from build123d import *

# Parameters (mm, degrees)
F0_W     = 10
F0_H     = 10
F3_DEPTH = 5
F1_W     = 10
F1_H     = 10
F4_DEPTH = 5
F2_W     = 10
F2_H     = 10
F5_DEPTH = 5


with BuildPart() as f3:
    # F0 (on Front) → F3 (new body, symmetric)
    with BuildSketch(Plane.XZ):
        Rectangle(F0_W, F0_H)
        Polygon((-4, 0), (0, 4), (4, 0), (0, -4), align=None, mode=Mode.SUBTRACT)
    extrude(amount=F3_DEPTH, both=True)

    # F1 (on Right) → F4 (intersect, symmetric)
    with BuildSketch(Plane.YZ):
        Rectangle(F1_W, F1_H)
        Polygon((-4, 0), (0, 4), (4, 0), (0, -4), align=None, mode=Mode.SUBTRACT)
    extrude(amount=F4_DEPTH, both=True, mode=Mode.INTERSECT)

    # F2 (on Top) → F5 (intersect, symmetric)
    with BuildSketch(Plane.XY):
        Rectangle(F2_W, F2_H)
        Polygon((-4, 0), (0, 4), (4, 0), (0, -4), align=None, mode=Mode.SUBTRACT)
    extrude(amount=F5_DEPTH, both=True, mode=Mode.INTERSECT)


solid = f3.part
Geometry check sheet. Reference: the model listing, model coordinates, mm. A direction names the side the tool comes from. Give positions to 0.01 mm unless a question says otherwise; leave off trailing zeros. Loops run counter-clockwise (first coordinate to the right, second up) from the corner with the lowest first, then second, coordinate; pieces in that order, holes last. Notation, with made-up numbers: M 73,41 L 131,41 A21 ccw 131,76 Z; hole C 34,-17 d5. An arc over 180 degrees is marked long. Answer as a JSON object with one key per item and string values. Group by question number.
Item 1: Sectioned sample at B-B on x = 0.25. Record the boundary of the cut face in (y, z).
Item 2: Sectioned sample at A-A on z = -2.5. Record the boundary of the cut face in (x, y), plus the area to 3 significant figures.
Item 3: Sectioned sample at D-D on y = 4.25. Record the boundary of the cut face in (x, z), plus the area to 3 significant figures.
Item 4: Sectioned sample at C-C on y = -1.5. Record the boundary of the cut face in (x, z).
Item 5: Material ranges on L1, parallel to Z at x = -4, y = 2; L2, parallel to Z at x = -3, y = -4.5, recorded low to high.
Item 6: Mould release check, pull along Z, two halves, no side actions. Record for faces 1 (the flat face through (-2, 4, -2)), 2 (the flat face through (-2.3, -2.3, -5)), 3 (the flat face through (-5, -2.3, -2.3)), 4 (the flat face through (4, 2, 2)): pulls with the +Z half, pulls with the -Z half, needs draft (parallel to the pull), parting line crosses it, or undercut.
Item 7: Gauge pin test, flat ends, axial feed: pin 1 (1.5 mm diameter, centred on x = 1, z = 2, fed in from -Y); pin 2 (1 mm diameter, centred on x = -1, z = 2, fed in from -Y). Record the tip position at first contact, or that the pin passes through.
Item 8: Access from +Z, -Z, +X, -X, +Y, -Y to the whole of each face (thin tool, end or side, straight path). Record for faces 5 (the flat face through (-2.3, -5, 2.3)), 6 (the flat face through (2, -4, 2)), 7 (the flat face through (2, 2, -4)), 8 (the flat face through (4, 2, -2)).
Findings below:
{
 "1": {"outline": "M -5,-5 L -3.75,-5 L -3.75,-3.75 L -5,-3.75 Z; M -5,3.75 L -3.75,3.75 L -3.75,5 L -5,5 Z; M 3.75,-5 L 5,-5 L 5,-3.75 L 3.75,-3.75 Z; M 3.75,3.75 L 5,3.75 L 5,5 L 3.75,5 Z"},
 "2": {"outline": "M -5,-5 L -1.5,-5 L -1.5,-2.5 L -2.5,-1.5 L -5,-1.5 Z; M -5,1.5 L -2.5,1.5 L -1.5,2.5 L -1.5,5 L -5,5 Z; M 1.5,-5 L 5,-5 L 5,-1.5 L 2.5,-1.5 L 1.5,-2.5 Z; M 1.5,2.5 L 2.5,1.5 L 5,1.5 L 5,5 L 1.5,5 Z", "area": "47.0 mm2"},
 "3": {"outline": "M -5,-5 L 5,-5 L 5,5 L -5,5 Z; hole M -4,0 L 0,-4 L 4,0 L 0,4 Z", "area": "68.0 mm2"},
 "4": {"outline": "M -5,-5 L -2.5,-5 L -2.5,-2.5 L -5,-2.5 Z; M -5,2.5 L -2.5,2.5 L -2.5,5 L -5,5 Z; M 2.5,-5 L 5,-5 L 5,-2.5 L 2.5,-2.5 Z; M 2.5,2.5 L 5,2.5 L 5,5 L 2.5,5 Z"},
 "5": {"L1": "-5 to -2, 2 to 5", "L2": "-5 to -1, 1 to 5"},
 "6": {"face 1": "undercut", "face 2": "pulls with the -Z half", "face 3": "needs draft", "face 4": "undercut"},
 "7": {"pin 1": "y = -5", "pin 2": "through"},
 "8": {"face 5": "+Z, -Z, +X, -X, -Y", "face 6": "+Y, -Y", "face 7": "+Z, -Z", "face 8": "+X, -X"}
}
